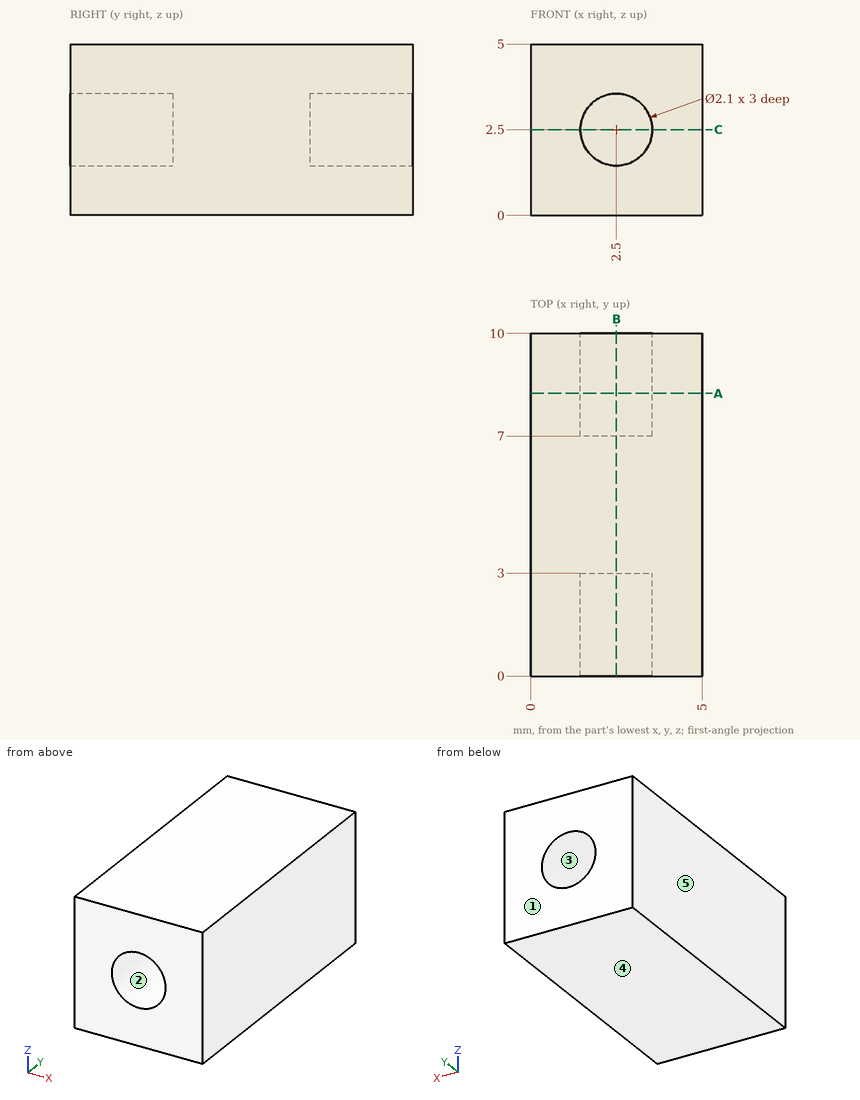
Input: dimensioned drawing with shaded views. Units: mm. Origin: part minimum x, y, z. A direction names the side the tool comes from. Coordinates: 2 decimals unless noted, no trailing zeros. Loops run counter-clockwise (first coordinate to the right, second up) from the corner with the lowest first, then second, coordinate; pieces in that order, holes last. Notation, with made-up numbers: (-5.75, 84.25) -> (33.25, 84.25) arc R14 cw to (33.25, 109.25) -> close; hole circle Ø11 at (71.5, 9). An arc over 180 degrees is marked (long way). Use a Markdown table: item, result. Add a question column.
(1) Section query B-B, the plane x = 2.5. Return loops of the section in (y, z), plus the area to 3 significant figures.
(2) Section query C-C, the plane z = 2.5. Return loops of the section in (x, y), plus the area to 3 significant figures.
(3) Access query for the marked faces 1 and 2. Directions: +Z, -Z, +X, -X, +Y, -Y. A direction counts if a zero-diameter tool reaches every point of the face in a straight line with its end or side. Return the directions, or none.
(4) Mould query, pull axis X, two halves, no side actions, for the marked faces 3, 4 and 5. Classes: pulls with the +X half, pulls with the -X half, needs draft (parallel to the pull), parting line crosses it, or undercut.
(5) Pin query (flat end, axial travel): pin 1 Ø2 at (y, z) = (6.5, 3) entering from -X; pin 2 Ø1 at (x, z) = (3, 2.5) entering from -Y; pin 3 Ø0.6 at (x, z) = (3, 2.5) entering from +Y. Return the tip coordinate at first contact, or that it passes through.
(6) Section query A-A, the plane y = 8.25. Return loops of the section in (x, z).
(7) Line query: line 1 along X through (y, z) = (1.75, 2.5); line 2 along Z through (x, y) = (3, 7.25); line 3 along Y through (x, z) = (1.65, 2.25). Output: solid intervals per line, ascending.
Answer:
| question | item | result |
|---|---|---|
| 1 | outline | (0, 0) -> (10, 0) -> (10, 1.45) -> (7, 1.45) -> (7, 3.55) -> (10, 3.55) -> (10, 5) -> (0, 5) -> (0, 3.55) -> (3, 3.55) -> (3, 1.45) -> (0, 1.45) -> close |
| 1 | area | 37.4 mm^2 |
| 2 | outline | (0, 0) -> (1.45, 0) -> (1.45, 3) -> (3.55, 3) -> (3.55, 0) -> (5, 0) -> (5, 10) -> (3.55, 10) -> (3.55, 7) -> (1.45, 7) -> (1.45, 10) -> (0, 10) -> close |
| 2 | area | 37.4 mm^2 |
| 3 | face 1 | +Z, -Z, +X, -X, +Y |
| 3 | face 2 | -Y |
| 4 | face 3 | undercut |
| 4 | face 4 | needs draft |
| 4 | face 5 | pulls with the -X half |
| 5 | pin 1 | stops at x = 0 |
| 5 | pin 2 | stops at y = 3 |
| 5 | pin 3 | stops at y = 7 |
| 6 | outline | (0, 0) -> (5, 0) -> (5, 5) -> (0, 5) -> close; hole circle Ø2.1 at (2.5, 2.5) |
| 7 | line 1 | x = 0 to 1.45, 3.55 to 5 |
| 7 | line 2 | z = 0 to 1.58, 3.42 to 5 |
| 7 | line 3 | y = 3 to 7 |
